Could you check a few things on this model? Use its own coordinates, in mm. A direction names the side the tool comes from. Give positions to 0.01 mm unless a question says otherwise; leave off trailing zeros. Write each loop counter-clockwise with the first axis right and the second up, starting at its lowest first coordinate (ties: lowest second). Pieces come first, ordered by that corner, then holes. Notation, with made-up numbers: (-28, -39) - (3, -39) arc R16 ccw to (3, -8) - close; hole circle Ø11 at (55.25, 12.25). An arc over 180 degrees is marked (long way). Answer as CSV lines item,"result". Start each with the question number.
Q1. Imagine slicing it at A-A on y = 0. List the corners of the cut face in (x, z) for me, and give its area (3 significant figures).
Q2. On a 3-axis mill with a long thin cutter (end or side, diameter ignored), from which of +Z, -Z, +X, -X, +Y, -Y can I reach the whole of each face in a straight line? I mean faces 5 (the face through (73.034, 16.946, -0.683)), 6 (the face through (-3, 0, -22.86)), 7 (the face through (-50.8, 24, 0)). Say none if no direction works.
Q3. If I drill on line 1 along Y through (x, z) = (72.75, 0) (3 decimals); line 2 along Z through (x, y) = (-30, -10.5), over which ranges is the centre line in solid material (lowest first)?
Q4. Will these pins go through, and if not, where does the flat tip stop? pin 1 Ø0.8 at (y, z) = (24.5, 5.5) entering from -X; pin 2 Ø2 at (y, z) = (-15.875, 0) entering from +X; pin 3 Ø1.5 at (y, z) = (-1, -14.5) entering from -X.
Q5. Imagine slicing it at B-B on x = 46.5. List the corners of the cut face in (y, z) for me.
Q6. Imagine slicing it at D-D on y = 6. List the corners of the cut face in (x, z) for me, and give its area (3 significant figures).
Q7. We'd pull the mould along Y, two halves only. Please class faces 1 (the face through (-50.8, -24, 0)), 2 (the face through (-53.98, 0.14, -24.15)), 3 (the face through (-3, 0, 22.86)), 4 (the face through (12, -25.4, 0)): pulls with the +Y half, pulls with the -Y half, needs draft (parallel to the pull), parting line crosses it, or undercut.
Q8. Imagine slicing it at C-C on z = 15.5. List the corners of the cut face in (x, y) for me.
```python
from build123d import *

# Parameters (mm, degrees)
SKETCH2_R           = 3.18135
BOSS_EXTRUDE1_DEPTH = 25.4
SKETCH5_W           = 45.72
SKETCH5_H           = 45.72
CUT_EXTRUDE1_DEPTH  = 72.39
SKETCH6_W           = 45.72
SKETCH6_H           = 45.72
CUT_EXTRUDE2_DEPTH  = 83.82
CUT_EXTRUDE3_REACH  = 151.86
SKETCH8_R           = 11.43
SKETCH8_R_2         = 1.27


with BuildPart() as part:
    # Sketch2 → Boss-Extrude1 (new body, symmetric)
    with BuildSketch(Plane.XY):
        with BuildLine():
            Line((-50.8, 25.4), (73.66, 25.4))
            Line((73.66, 25.4), (73.66, -25.4))
            Line((73.66, -25.4), (-50.8, -25.4))
            ThreePointArc((-50.8, -25.4), (-76.2, 0), (-50.8, 25.4))
        make_face()
        with Locations((-50.8, 0)):
            Circle(SKETCH2_R, mode=Mode.SUBTRACT)
    extrude(amount=BOSS_EXTRUDE1_DEPTH, both=True)

    # Sketch5 → Cut-Extrude1 (cut, symmetric)
    with BuildSketch(Plane(origin=(0, 0, 0), x_dir=(0, 0, -1), z_dir=(1, 0, 0))):
        Rectangle(SKETCH5_W, SKETCH5_H)
    extrude(amount=CUT_EXTRUDE1_DEPTH, both=True, mode=Mode.SUBTRACT)

    # Sketch6 → Cut-Extrude2 (cut, symmetric)
    with BuildSketch(Plane(origin=(0, 0, 0), x_dir=(1, 0, 0), z_dir=(0, 1, 0))):
        with Locations((-73.66, 0)):
            Rectangle(SKETCH6_W, SKETCH6_H)
    extrude(amount=CUT_EXTRUDE2_DEPTH, both=True, mode=Mode.SUBTRACT)

    # Sketch8 → Cut-Extrude3 (cut, up to next)
    with BuildSketch(Plane(origin=(73.66, 0, 0), x_dir=(0, 0, -1), z_dir=(1, 0, 0)), mode=Mode.PRIVATE) as cut_extrude3_sk1:
        Circle(SKETCH8_R)
    cut_extrude3_tool1 = extrude(cut_extrude3_sk1.sketch, amount=-CUT_EXTRUDE3_REACH, mode=Mode.PRIVATE) & part.part
    add(cut_extrude3_tool1.solids().sort_by_distance((73.66, 0, 0))[0], mode=Mode.SUBTRACT)
    # Sketch8 → Cut-Extrude3 (cut, up to next)
    with BuildSketch(Plane(origin=(73.66, 0, 0), x_dir=(0, 0, -1), z_dir=(1, 0, 0)), mode=Mode.PRIVATE) as cut_extrude3_sk2:
        with Locations((0, 15.875)):
            Circle(SKETCH8_R_2)
    cut_extrude3_tool2 = extrude(cut_extrude3_sk2.sketch, amount=-CUT_EXTRUDE3_REACH, mode=Mode.PRIVATE) & part.part
    add(cut_extrude3_tool2.solids().sort_by_distance((73.66, 15.875, 0))[0], mode=Mode.SUBTRACT)
    # Sketch8 → Cut-Extrude3 (cut, up to next)
    with BuildSketch(Plane(origin=(73.66, 0, 0), x_dir=(0, 0, -1), z_dir=(1, 0, 0)), mode=Mode.PRIVATE) as cut_extrude3_sk3:
        with Locations((0, -15.875)):
            Circle(SKETCH8_R_2)
    cut_extrude3_tool3 = extrude(cut_extrude3_sk3.sketch, amount=-CUT_EXTRUDE3_REACH, mode=Mode.PRIVATE) & part.part
    add(cut_extrude3_tool3.solids().sort_by_distance((73.66, -15.875, 0))[0], mode=Mode.SUBTRACT)


solid = part.part
```
Conclusion:
1,outline,"(-76.2, -25.4) - (-53.98, -25.4) - (-53.98, -22.86) - (-76.2, -22.86) - close; (-76.2, 22.86) - (-53.98, 22.86) - (-53.98, 25.4) - (-76.2, 25.4) - close; (-47.62, -25.4) - (73.66, -25.4) - (73.66, -11.43) - (72.39, -11.43) - (72.39, -22.86) - (-47.62, -22.86) - close; (-47.62, 22.86) - (72.39, 22.86) - (72.39, 11.43) - (73.66, 11.43) - (73.66, 25.4) - (-47.62, 25.4) - close"
1,area,"758 mm^2"
2,face 5,"+X, -X"
2,face 6,"-X"
2,face 7,"-X, +Y, -Y"
3,line 1,"-25.4 to -17.145, -14.605 to -11.43, 11.43 to 14.605, 17.145 to 25.4"
3,line 2,"-25.4 to -22.86, 22.86 to 25.4"
4,pin 1,"x = -50.8"
4,pin 2,"through"
4,pin 3,"x = 72.39"
5,outline,"(-25.4, -25.4) - (25.4, -25.4) - (25.4, 25.4) - (-25.4, 25.4) - close; hole (-22.86, -22.86) - (22.86, -22.86) - (22.86, 22.86) - (-22.86, 22.86) - close"
6,outline,"(-75.48, -25.4) - (73.66, -25.4) - (73.66, -9.73) - (72.39, -9.73) - (72.39, -22.86) - (-75.48, -22.86) - close; (-75.48, 22.86) - (72.39, 22.86) - (72.39, 9.73) - (73.66, 9.73) - (73.66, 25.4) - (-75.48, 25.4) - close"
6,area,"791 mm^2"
7,face 1,"needs draft"
7,face 2,"undercut"
7,face 3,"undercut"
7,face 4,"pulls with the -Y half"
8,outline,"(-50.8, -25.4) - (73.66, -25.4) - (73.66, 25.4) - (-50.8, 25.4) - (-50.8, 22.86) - (72.39, 22.86) - (72.39, -22.86) - (-50.8, -22.86) - close"
